For this review, use the dimensioned drawing (mm, ordinates from the lowest corner) and the shaded views. A direction names the side the tool comes from. Give positions to 0.01 mm unless a question says otherwise; leave off trailing zeros. Loops run counter-clockwise (first coordinate to the right, second up) from the corner with the lowest first, then second, coordinate; pieces in that order, holes last. Notation, with made-up numbers: (7, 88) -> (46, 88) arc R35 cw to (46, 125) -> close; hole circle Ø8 at (64.5, 75.25). An arc over 180 degrees is marked (long way). Use a Markdown table: item, result. Add a question column.
1. To check wall thickness, follow line 1 (X direction, y = 2.5, z = 21); line 2 (Y direction, x = 13.5, z = 13). State the ranges of each line that lie inside material, in increasing order.
2. For the marked faces 1, 2 and 3, list the 3-axis set-ups (+Z, -Z, +X, -X, +Y, -Y) from which the entire face can be reached by the end or side of a thin tool; tool diameter is ignored.
3. Add section A-A (y = 25.5). State the section outline as (x, z) points, and give its area (3 significant figures).
4. For pin 1 Ø1 at (x, z) = (7, 5) entering from +Y; pin 2 Ø15 at (x, z) = (21.5, 10.5) entering from +Y, all flat-tipped, find the tip position at first contact; note any pin that passes through.
5. Add section B-B (z = 21). State the section outline as (x, y) points, and give its area (3 significant figures).
6. Add section C-C (x = 25). State the section outline as (y, z) points.
7. Add section D-D (y = 12.5). State the section outline as (x, z) points, and give its area (3 significant figures).
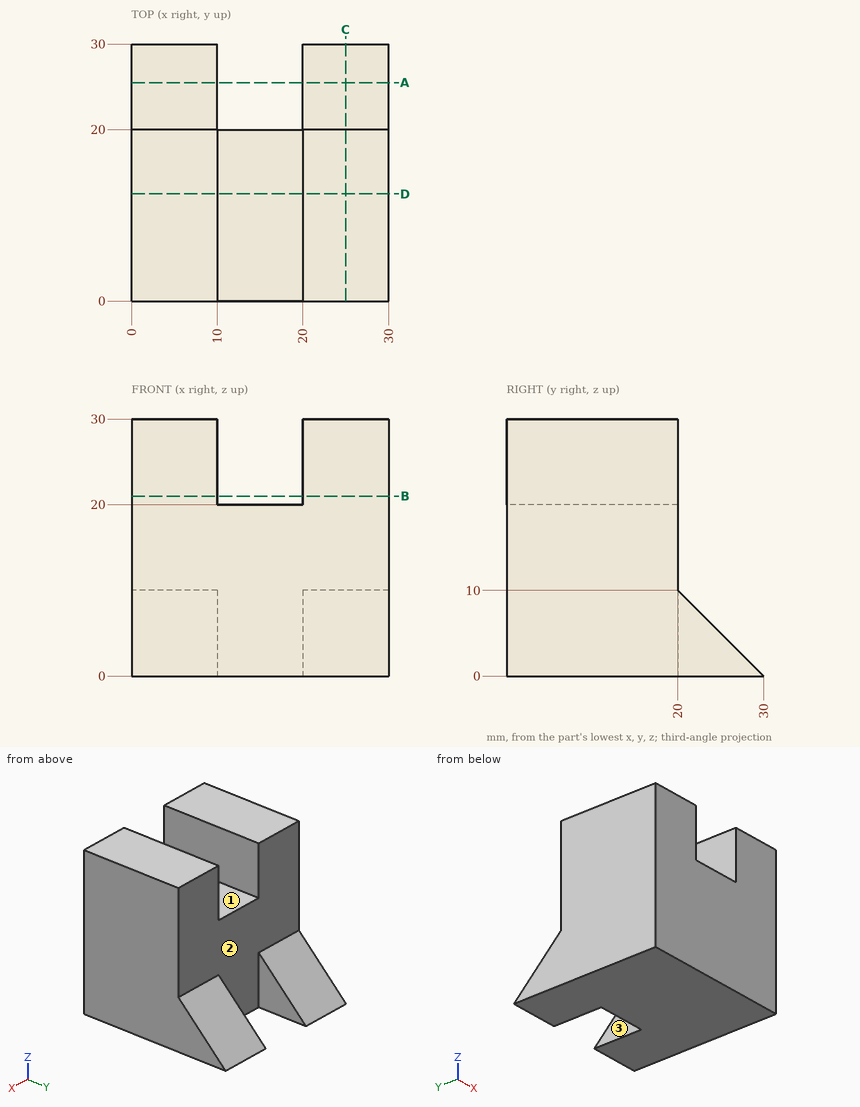
Taken from the geometry:
| question | item | result |
|---|---|---|
| 1 | line 1 | x = 0 to 10, 20 to 30 |
| 1 | line 2 | y = 0 to 20 |
| 2 | face 1 | +Z, +Y, -Y |
| 2 | face 2 | +Z, +Y |
| 2 | face 3 | +Z, -Z, +Y |
| 3 | outline | (0, 0) -> (10, 0) -> (10, 4.5) -> (0, 4.5) -> close; (20, 0) -> (30, 0) -> (30, 4.5) -> (20, 4.5) -> close |
| 3 | area | 90.0 mm^2 |
| 4 | pin 1 | stops at y = 25.5 |
| 4 | pin 2 | stops at y = 27 |
| 5 | outline | (0, 0) -> (10, 0) -> (10, 20) -> (0, 20) -> close; (20, 0) -> (30, 0) -> (30, 20) -> (20, 20) -> close |
| 5 | area | 400 mm^2 |
| 6 | outline | (0, 0) -> (30, 0) -> (20, 10) -> (20, 30) -> (0, 30) -> close |
| 7 | outline | (0, 0) -> (30, 0) -> (30, 30) -> (20, 30) -> (20, 20) -> (10, 20) -> (10, 30) -> (0, 30) -> close |
| 7 | area | 800 mm^2 |
